Here's how the part is built. I have some questions about the finished solid (model axes, mm). Face numbers are marked on the shaded views. A direction names the side the tool comes from. Round coordinates to 2 decimals unless told otherwise and drop trailing zeros. Order: outer loops, then holes, each group sorted by start corner. A loop starts at its lowest first (then second) coordinate and runs counter-clockwise, first axis right, second up. Notation, with made-up numbers: (-5, 45) - (10, 45) arc R11 ccw to (10, 55) - close; hole circle Ø3 at (62.25, 32). An arc over 180 degrees is marked (long way). Answer as a JSON object with one key per item and string values.
Autodesk Inventor part; units mm, degrees
ref_plane "YZ Plane" through (0, 0, 0) normal (1, 0, 0) x (0, 1, 0)
ref_plane "XZ Plane" through (0, 0, 0) normal (0, 1, 0) x (-1, 0, 0)
ref_plane "XY Plane" through (0, 0, 0) normal (0, 0, 1) x (1, 0, 0)
sketch "Sketch_1" plane through (0, 0, 0) normal (0, 0, 1) x (1, 0, 0)
  arc A0 (-19.05, 3.175) -> (-15.875, 0) centre (-15.875, 3.175) ccw
  line L0 (-15.875, 0) -> (15.875, 0)
  arc A1 (15.875, 0) -> (19.05, 3.175) centre (15.875, 3.175) ccw
  line L1 (19.05, 3.175) -> (19.05, 15.875)
  arc A2 (19.05, 15.875) -> (15.875, 19.05) centre (15.875, 15.875) ccw
  line L2 (15.875, 19.05) -> (5.6388, 19.05)
  arc A3 (5.6388, 19.05) -> (4.064, 17.4752) centre (5.6388, 17.4752) ccw
  line L3 (4.064, 17.4752) -> (4.064, 16.5608)
  arc A4 (4.064, 16.5608) -> (5.6388, 14.986) centre (5.6388, 16.5608) ccw
  line L4 (5.6388, 14.986) -> (9.398, 14.986)
  arc A5 (10.287, 14.097) -> (9.398, 14.986) centre (9.398, 14.097) ccw
  line L5 (10.287, 14.097) -> (10.287, 13.7794)
  arc A6 (10.0266, 13.1508) -> (10.287, 13.7794) centre (9.398, 13.7794) ccw
  line L6 (10.0266, 13.1508) -> (5.125, 8.2492)
  arc A7 (1.7664, 6.858) -> (5.125, 8.2492) centre (1.7664, 11.6078) ccw
  line L7 (1.7664, 6.858) -> (-1.7664, 6.858)
  arc A8 (-5.125, 8.2492) -> (-1.7664, 6.858) centre (-1.7664, 11.6078) ccw
  line L8 (-5.125, 8.2492) -> (-10.0266, 13.1508)
  arc A9 (-10.287, 13.7794) -> (-10.0266, 13.1508) centre (-9.398, 13.7794) ccw
  line L9 (-10.287, 13.7794) -> (-10.287, 14.097)
  arc A10 (-9.398, 14.986) -> (-10.287, 14.097) centre (-9.398, 14.097) ccw
  line L10 (-9.398, 14.986) -> (-5.6388, 14.986)
  arc A11 (-5.6388, 14.986) -> (-4.064, 16.5608) centre (-5.6388, 16.5608) ccw
  line L11 (-4.064, 16.5608) -> (-4.064, 17.4752)
  arc A12 (-4.064, 17.4752) -> (-5.6388, 19.05) centre (-5.6388, 17.4752) ccw
  line L12 (-5.6388, 19.05) -> (-15.875, 19.05)
  arc A13 (-15.875, 19.05) -> (-19.05, 15.875) centre (-15.875, 15.875) ccw
  line L13 (-19.05, 15.875) -> (-19.05, 3.175)
  circle A14 centre (14.8488, 14.8014) radius 2.5527
  circle A15 centre (12.7, 6.35) radius 3.3274
  circle A16 centre (-12.7, 6.35) radius 3.3274
  circle A17 centre (-14.8488, 14.8014) radius 2.5527
extrude "Extrusion1" add sketch "Sketch_1" against normal blind 50.8
properties part number "1575-2-CL"
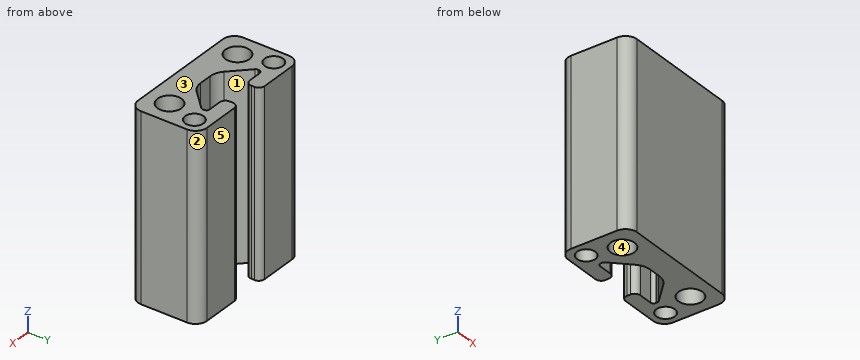
1. Imagine slicing it at C-C (z = -32). Give the number of separate pieces and of enclosed holes in the cut face, plus the area to 3 significant figures.
Responses:
{"separate pieces": "1", "enclosed holes": "4", "area": "449 mm2"}
2. Imagine slicing it at B-B (x = -6.5). List the corners of the cut face in (y, z) for me, plus the area to 3 significant figures.
Responses:
{"outline": "(0, -50.8) - (9.62, -50.8) - (9.62, 0) - (0, 0) - close; (14.99, -50.8) - (19.05, -50.8) - (19.05, 0) - (14.99, 0) - close", "area": "695 mm2"}
3. For the marked faces 1 and 2, which set-ups out of +Z, -Z, +X, -X, +Y, -Y let a thin tool reach every point of the face, with its end or its side?
Responses:
{"face 1": "+Z, -Z", "face 2": "+Z, -Z, +X, +Y"}
4. Imagine slicing it at D-D (y = 5.75). List the corners of the cut face in (x, z) for me, plus the area to 3 significant figures.
Responses:
{"outline": "(-19.05, -50.8) - (-15.97, -50.8) - (-15.97, 0) - (-19.05, 0) - close; (-9.43, -50.8) - (9.43, -50.8) - (9.43, 0) - (-9.43, 0) - close; (15.97, -50.8) - (19.05, -50.8) - (19.05, 0) - (15.97, 0) - close", "area": "1,270 mm2"}
5. If I drill on L1, parallel to X at y = 5.25, z = -46.5; L2, parallel to X at y = 5.5, z = -26; L3, parallel to Y at x = 13, z = -22.5, over which ranges is the centre line in solid material (lowest first)? Write a range as [from, to].
Responses:
{"L1": "[-19.05, -15.84], [-9.56, 9.56], [15.84, 19.05]", "L2": "[-19.05, -15.92], [-9.48, 9.48], [15.92, 19.05]", "L3": "[0, 3.04], [9.66, 13.04], [16.56, 19.05]"}
6. For P1, Ø0.5, axis at y = 17, z = -28, coming from the +X side; P2, Ø1.8, axis at x = 0, z = -32.5, coming from the +Y side; P3, Ø1, axis at y = 17, z = -41.5, coming from the +X side, each with a flat end and sliding along its axis, tell me the tip position at first contact or that it passes through.
Responses:
{"P1": "x = 18.93", "P2": "y = 6.86", "P3": "x = 18.99"}
7. Thinking about a two-plate mould opening in Y: for the marked faces 3, 4 and 5, which applies, pulls with the +Y half, pulls with the -Y half, needs draft (parallel to the pull), parting line crosses it, or undercut?
Responses:
{"face 3": "needs draft", "face 4": "undercut", "face 5": "pulls with the +Y half"}
8. Imagine slicing it at A-A (y = 10.25). List the corners of the cut face in (x, z) for me, plus the area to 3 significant figures.
Responses:
{"outline": "(-19.05, -50.8) - (-7.13, -50.8) - (-7.13, 0) - (-19.05, 0) - close; (7.13, -50.8) - (19.05, -50.8) - (19.05, 0) - (7.13, 0) - close", "area": "1,210 mm2"}
